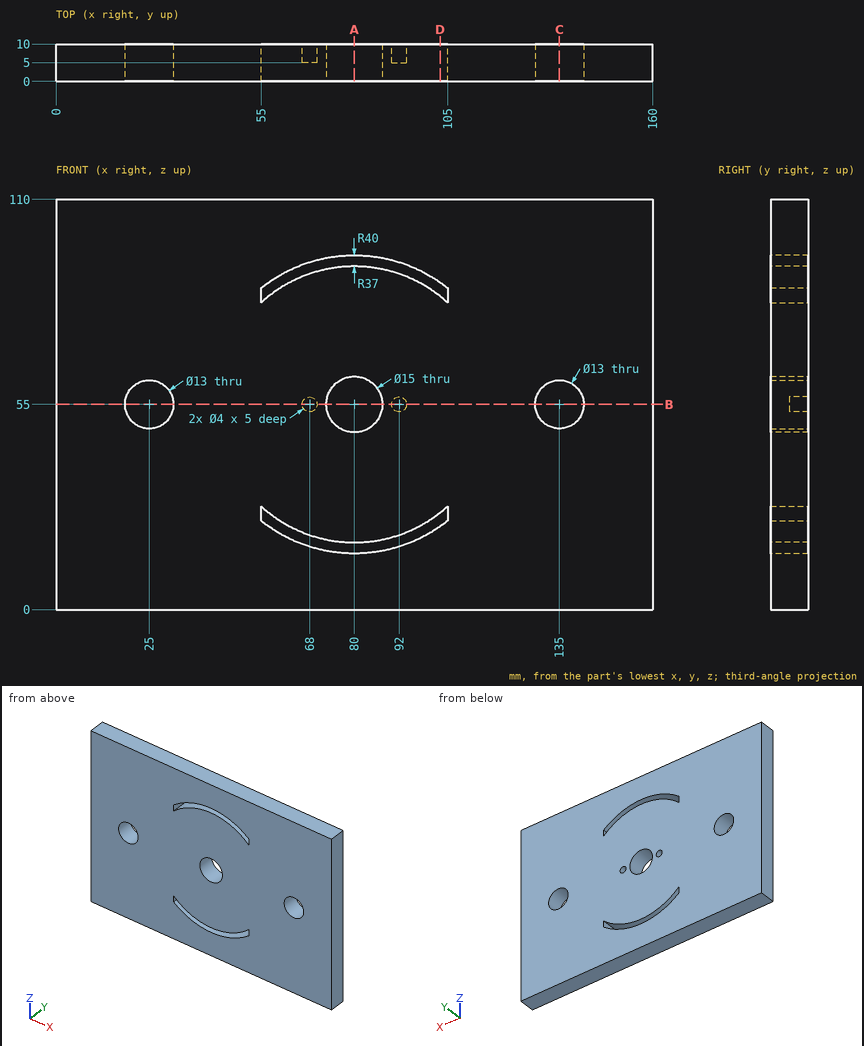
The drawing under review shows one solid part. Ordinate dimensions are in mm from its lowest x, y, z. Round coordinates to 2 decimals unless told otherwise and drop trailing zeros. Write each loop counter-clockwise with the first axis right and the second up, starting at its lowest first coordinate (ties: lowest second). Pieces come first, ordered by that corner, then holes. Notation, with made-up numbers: (68, -4) -> (116, -4) arc R27 cw to (116, 30) -> close; hole circle Ø6 at (68, 70). An arc over 180 degrees is marked (long way). Put each result on its own line as item: value.
Q1. Clearance check with a flat-ended pin moving along its axis: pin 1 Ø1.2 at (x, z) = (91.5, 55.5) entering from +Y. State where the tip first meets the part, or that it passes through.
Determined:
pin 1: stops at y = 5
Q2. Consider section A-A on x = 80. State the section outline as (y, z) points, and give its area (3 significant figures).
Determined:
outline: (0, 0) -> (10, 0) -> (10, 15) -> (0, 15) -> close; (0, 18) -> (10, 18) -> (10, 47.5) -> (0, 47.5) -> close; (0, 62.5) -> (10, 62.5) -> (10, 92) -> (0, 92) -> close; (0, 95) -> (10, 95) -> (10, 110) -> (0, 110) -> close
area: 890 mm^2
Q3. Consider section D-D on x = 103. State the section outline as (y, z) points, and give its area (3 significant figures).
Determined:
outline: (0, 0) -> (10, 0) -> (10, 22.27) -> (0, 22.27) -> close; (0, 26.02) -> (10, 26.02) -> (10, 83.98) -> (0, 83.98) -> close; (0, 87.73) -> (10, 87.73) -> (10, 110) -> (0, 110) -> close
area: 1,030 mm^2
Q4. Consider section B-B on z = 55. State the section outline as (x, y) points.
Determined:
outline: (0, 0) -> (18.5, 0) -> (18.5, 10) -> (0, 10) -> close; (31.5, 0) -> (72.5, 0) -> (72.5, 10) -> (70, 10) -> (70, 5) -> (66, 5) -> (66, 10) -> (31.5, 10) -> close; (87.5, 0) -> (128.5, 0) -> (128.5, 10) -> (94, 10) -> (94, 5) -> (90, 5) -> (90, 10) -> (87.5, 10) -> close; (141.5, 0) -> (160, 0) -> (160, 10) -> (141.5, 10) -> close
Q5. To check wall thickness, follow L1, parallel to X at y = 2.25, z = 55; L2, parallel to Z at x = 92, y = 8.35; L3, parallel to Z at x = 135, y = 3. State the ranges of each line that lie inside material, in increasing order. Write a range as [from, to].
Determined:
L1: x = [0, 18.5], [31.5, 72.5], [87.5, 128.5], [141.5, 160]
L2: z = [0, 16.84], [20, 53], [57, 90], [93.16, 110]
L3: z = [0, 48.5], [61.5, 110]
Q6. Consider section C-C on x = 135. State the section outline as (y, z) points, and give its area (3 significant figures).
Determined:
outline: (0, 0) -> (10, 0) -> (10, 48.5) -> (0, 48.5) -> close; (0, 61.5) -> (10, 61.5) -> (10, 110) -> (0, 110) -> close
area: 970 mm^2
